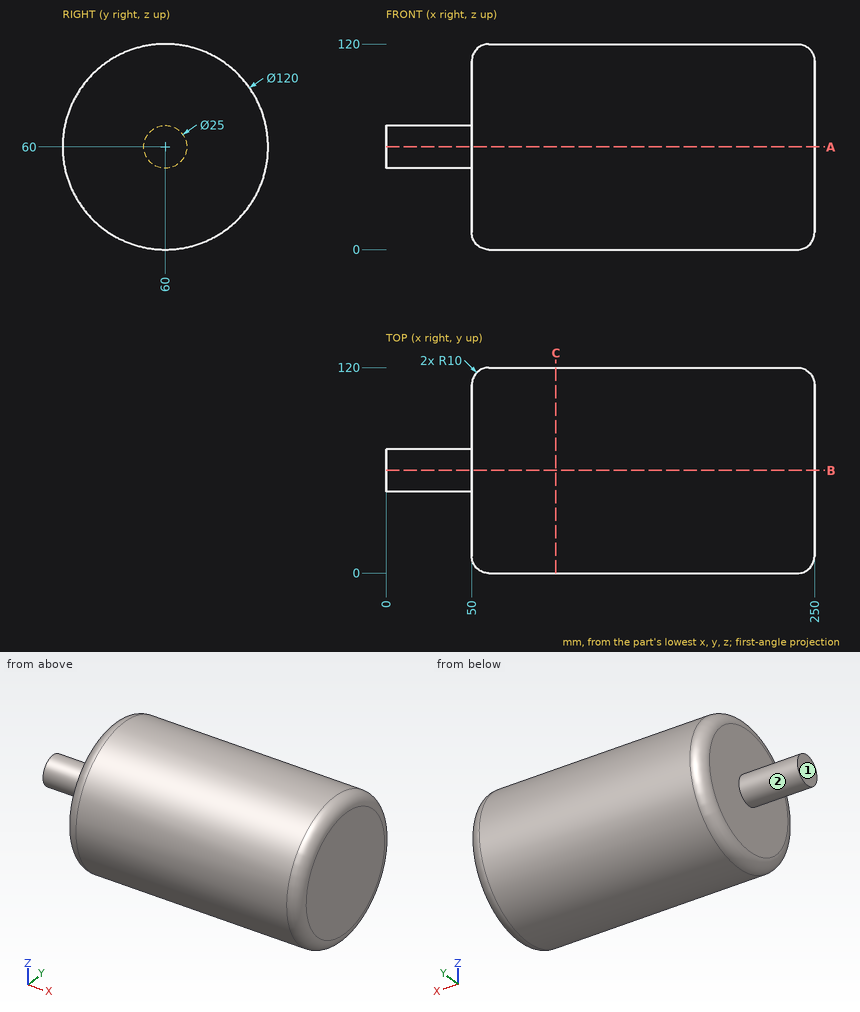
Geometry check sheet. Reference: drawing and pictorial views, mm from the part's lowest x, y, z. A direction names the side the tool comes from. Coordinates: 2 decimals unless noted, no trailing zeros. Order: outer loops, then holes, each group sorted by start corner. A loop starts at its lowest first (then second) coordinate and runs counter-clockwise, first axis right, second up.
Item 1: Section check C-C (x = 99). Enter the section's corners in (y, z).
Item 2: Tool access check on the marked faces 1 and 2. Record the directions out of +Z, -Z, +X, -X, +Y, -Y that give a thin tool (end or side, any length) a straight path to the whole face; none if there is none.
Item 3: Section check A-A (z = 60). Enter the section's corners in (x, y), plus the area to 3 significant figures.
Item 4: Depth check by flat-ended pin: pin 1 (6 mm diameter, centred on x = 74, y = 71, fed in from -Z); pin 2 (2 mm diameter, centred on x = 146.5, y = 13.5, fed in from -Z); pin 3 (5 mm diameter, centred on x = 37.5, z = 72.5, fed in from -Y); pin 4 (8 mm diameter, centred on x = 45, y = 17, fed in from -Z). Enter the tip coordinate at first touch or a pass-through.
Item 5: Scan lines: line 1 along X through (y, z) = (94, 46); line 2 along Z through (x, y) = (172, 62). Record each from-to range of solid material in increasing order.
Check sheet entries:
1. outline: circle Ø120 at (60, 60)
2. face 1: +Z, -Z, -X, +Y, -Y
2. face 2: -X
3. outline: (0, 47.5) - (50, 47.5) - (50, 10) arc R10 ccw to (60, 0) - (240, 0) arc R10 ccw to (250, 10) - (250, 110) arc R10 ccw to (240, 120) - (60, 120) arc R10 ccw to (50, 110) - (50, 72.5) - (0, 72.5) - close
3. area: 25,200 mm2
4. pin 1: stops at z = 0.54
4. pin 2: stops at z = 20.89
4. pin 3: stops at y = 52.5
4. pin 4: passes through
5. line 1: x = 50 to 250
5. line 2: z = 0.03 to 119.97
